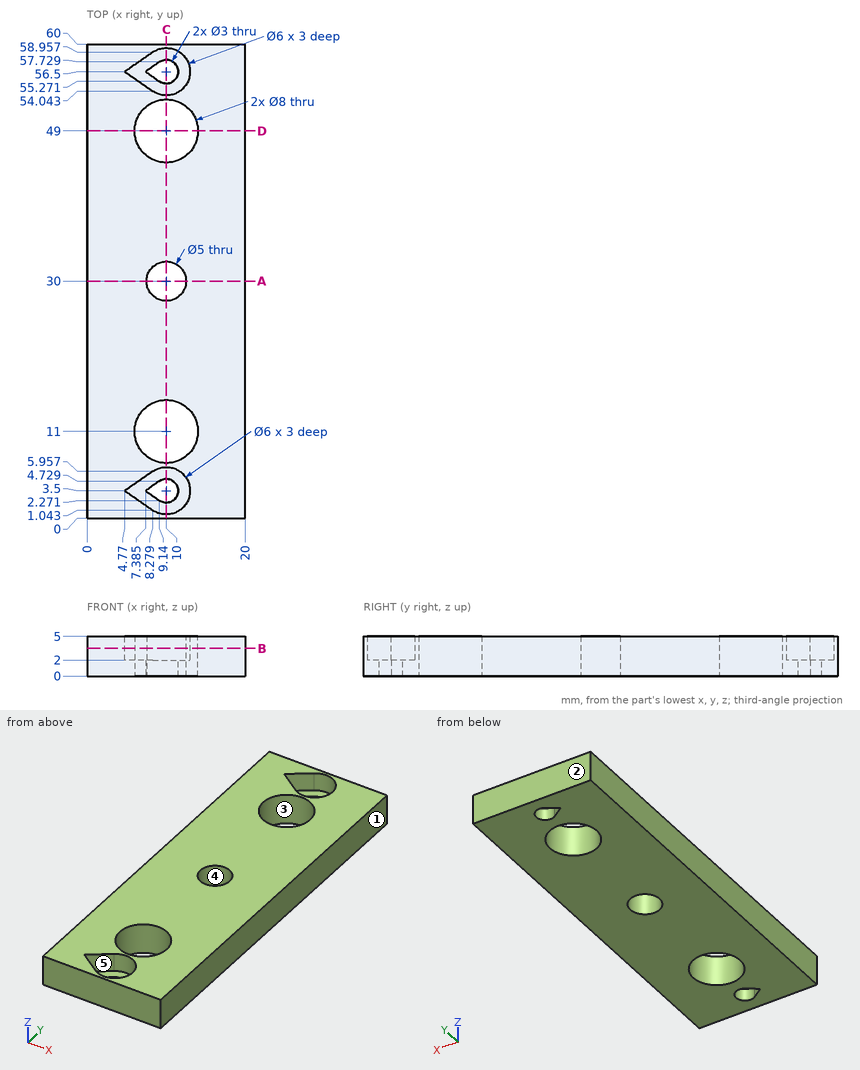
Can you work these out from the drawing? Everything is in mm from the part's minimum corner. A direction names the side the tool comes from. Round coordinates to 2 decimals unless told otherwise and drop trailing zeros. Loops run counter-clockwise (first coordinate to the right, second up) from the corner with the lowest first, then second, coordinate; pieces in that order, holes last.
1. We'd pull the mould along X, two halves only. Please class the marked faces 1, 2 and 3: +X half, -X half, draft (parallel to the pull), parting line (faces both ways), or undercut.
Answer list:
face 1: +X half
face 2: draft
face 3: undercut
2. If I drill on line 1 along Y through (x, z) = (10, 2.95); line 2 along Y through (x, z) = (10, 1.15); line 3 along X through (y, z) = (11, 2.7), over which ranges is the centre line in solid material (lowest first)?
Answer list:
line 1: y = 0 to 0.5, 6.5 to 7, 15 to 27.5, 32.5 to 45, 53 to 53.5, 59.5 to 60
line 2: y = 0 to 2, 5 to 7, 15 to 27.5, 32.5 to 45, 53 to 55, 58 to 60
line 3: x = 0 to 6, 14 to 20
3. If we section it at B-B on z = 3.5: Write out the boundary of the cut face in (x, y).
Answer list:
outline: (0, 0) - (20, 0) - (20, 60) - (0, 60) - close; hole (4.77, 3.5) - (8.28, 1.04) arc R3 ccw (long way) to (8.28, 5.96) - close; hole (4.77, 56.5) - (8.28, 54.04) arc R3 ccw (long way) to (8.28, 58.96) - close; hole circle Ø8 at (10, 11); hole circle Ø8 at (10, 49); hole circle Ø5 at (10, 30)
4. If we section it at C-C on x = 10: Count the separate pieces of the cut face and the enclosed holes in it, plus the area to 3 significant figures.
Answer list:
separate pieces: 6
enclosed holes: 0
area: 147 mm2
5. Which directions (+Z, -Z, +X, -X, +Y, -Y) give clear straight access to the entire face, cutting with the end or side of a thin tool? Please do the marked faces 4 and 5.
Answer list:
face 4: +Z, -Z
face 5: +Z
6. For P1, Ø5, axis at x = 10, y = 3.5, coming from the +Z side, with a flat end and sliding along its axis, tell me the tip position at first contact or that it passes through.
Answer list:
P1: stops at z = 2
7. If we section it at D-D on y = 49: Write out the boundary of the cut face in (x, z).
Answer list:
outline: (0, 0) - (6, 0) - (6, 5) - (0, 5) - close; (14, 0) - (20, 0) - (20, 5) - (14, 5) - close
8. If we section it at A-A on y = 30: Write out the boundary of the cut face in (x, z).
Answer list:
outline: (0, 0) - (7.5, 0) - (7.5, 5) - (0, 5) - close; (12.5, 0) - (20, 0) - (20, 5) - (12.5, 5) - close
